```python
from build123d import *

# Parameters (mm, degrees)
SKETCH1_W               = 28
SKETCH1_H               = 16
SKETCH1_W_2             = 22.6
SKETCH1_H_2             = 11.84
BOSS_EXTRUDE1_DEPTH     = 3
BOSS_EXTRU_1_DEPTH      = 5
BOSS_EXTRU_1_DEPTH_BACK = 18
ESQUISSE6_R             = 2
BOSS_EXTRU_3_DEPTH      = 17.7
ESQUISSE7_R             = 1
ENL_V_MAT_EXTRU_3_DEPTH = 4
ESQUISSE8_W             = 11.84
ESQUISSE8_H             = 2.37
ENL_V_MAT_EXTRU_4_DEPTH = 10
CONG_1_R                = 1
CONG_3_R                = 5
CONG_4_R                = 2.5
BOSS_EXTRUDE2_DEPTH     = 23


with BuildPart() as part:
    # Sketch1 → Boss-Extrude1 (new body)
    with BuildSketch(Plane(origin=(0, 0, 0), x_dir=(1, 0, 0), z_dir=(0, 1, 0))):
        with Locations((14, 8)):
            Rectangle(SKETCH1_W, SKETCH1_H)
        with Locations((15.8, 8)):
            Rectangle(SKETCH1_W_2, SKETCH1_H_2, mode=Mode.SUBTRACT)
    extrude(amount=BOSS_EXTRUDE1_DEPTH)

    # Esquisse1 → Boss.-Extru.1 (add, two sides: drawn at the far end of the back side and taken through both)
    with BuildSketch(Plane.XY.offset(-BOSS_EXTRU_1_DEPTH_BACK)):
        Polygon((34.226941016, 3), (35.226941016, -1), (62.4, -1), (62.4, -4), (33.4, -4), (32.4, 0), (28, 0), (28, 3), align=None)
    extrude(amount=BOSS_EXTRU_1_DEPTH + BOSS_EXTRU_1_DEPTH_BACK)

    # Esquisse6 → Boss.-Extru.3 (add)
    with BuildSketch(Plane(origin=(0, 3, 0), x_dir=(1, 0, 0), z_dir=(0, 1, 0))):
        with Locations(Location((31.113470508, 0, 0), (0, 0, 90))):
            Circle(ESQUISSE6_R)
        with Locations(Location((31.113470508, 16, 0), (0, 0, 90))):
            Circle(ESQUISSE6_R)
    extrude(amount=BOSS_EXTRU_3_DEPTH)

    # Esquisse7 → Enlèv. mat.-Extru.3 (cut)
    with BuildSketch(Plane(origin=(0, 20.7, 0), x_dir=(1, 0, 0), z_dir=(0, 1, 0))):
        with Locations(Location((31.113470508, 16, 0), (0, 0, 270))):
            Circle(ESQUISSE7_R)
        with Locations(Location((31.113470508, 0, 0), (0, 0, 270))):
            Circle(ESQUISSE7_R)
    extrude(amount=-ENL_V_MAT_EXTRU_3_DEPTH, mode=Mode.SUBTRACT)

    # Esquisse8 → Enlèv. mat.-Extru.4 (cut)
    with BuildSketch(Plane(origin=(0, -1, 0), x_dir=(1, 0, 0), z_dir=(0, 1, 0))):
        with Locations((41.52, 12.315)):
            Rectangle(ESQUISSE8_W, ESQUISSE8_H)
    extrude(amount=-ENL_V_MAT_EXTRU_4_DEPTH, mode=Mode.SUBTRACT)

    # Congé1
    cong_1_edges = [part.edges().sort_by_distance(p)[0] for p in [
        (28, 1.5, -16),
    ]]
    fillet(cong_1_edges, radius=CONG_1_R)
    cong_1_2_edges = [part.edges().sort_by_distance(p)[0] for p in [
        (28, 1.5, -18),
    ]]
    fillet(cong_1_2_edges, radius=CONG_1_R - 0.0001)  # a hair under: the kernel refuses the full size

    # Congé3
    cong_3_edges = [part.edges().sort_by_distance(p)[0] for p in [
        (0, 1.5, 0),
        (0, 1.5, -16),
    ]]
    fillet(cong_3_edges, radius=CONG_3_R)

    # Congé4
    cong_4_edges = [part.edges().sort_by_distance(p)[0] for p in [
        (28, 1.5, 0),
    ]]
    fillet(cong_4_edges, radius=CONG_4_R)
    cong_4_2_edges = [part.edges().sort_by_distance(p)[0] for p in [
        (28, 1.5, 5),
    ]]
    fillet(cong_4_2_edges, radius=CONG_4_R - 0.0001)  # a hair under: the kernel refuses the full size

    # Sketch3 → Boss-Extrude2 (add)
    with BuildSketch(Plane.XY.offset(5)):
        with BuildLine():
            Line((62.4, -1), (62.4, -4))
            Line((62.4, -4), (79.480551105, -4))
            ThreePointArc((79.480551105, -4), (85.080447122, -1.680447122), (87.4, 3.919448895))
            Line((87.4, 3.919448895), (87.4, 5.5))
            ThreePointArc((87.4, 5.5), (85.9, 7), (84.4, 5.5))
            Line((84.4, 5.5), (84.4, 3.919448895))
            ThreePointArc((84.4, 3.919448895), (83.315910874, 0.78923852), (80.528063722, -1))
            Line((80.528063722, -1), (79.4, -1))
            Line((79.4, -1), (71.856339273, -1))
            Line((71.856339273, -1), (62.4, -1))
        make_face()
    extrude(amount=-BOSS_EXTRUDE2_DEPTH)


solid = part.part
```
Source: CAD feature listing. Evaluate the final solid. Frame: model axes, mm. A direction names the side the tool comes from. Coordinates: 2 decimals unless noted, no trailing zeros. Write each loop counter-clockwise with the first axis right and the second up, starting at its lowest first coordinate (ties: lowest second). Pieces come first, ordered by that corner, then holes. Notation, with made-up numbers: (74.25, 59.25) -> (119.25, 59.25) arc R16 ccw to (119.25, 77.25) -> close; hole circle Ø9 at (-18, -35). An arc over 180 degrees is marked (long way). Return JSON: item names as keys, results as strings. Group by question number.
1) Section query B-B, the plane y = 1.75. State how many separate pieces and enclosed holes the cut face has, plus the area to 3 significant figures.
2) Section query C-C, the plane z = -3.5. Return loops of the section in (x, y).
3) Section query A-A, the plane z = -9.5. Return loops of the section in (x, y).
4) Section query D-D, the plane y = 8. Return loops of the section in (x, z).
5) Mould query, pull axis Z, two halves, no side actions, for faces 4 (the face through (1, 2, -2)), 5 (the face through (85.02, -1.74, -6.34)), 6 (the face through (41, -2, -13.5)). Classes: +Z half, -Z half, draft (parallel to the pull), parting line (faces both ways), or undercut.
6) Contact query for flat-ended pins moving along their axis: P1, Ø6, axis at x = 73.5, z = -9.5, coming from the +Y side; P2, Ø1.9, axis at y = -2, z = -12, coming from the -X side; P3, Ø11.5, axis at x = 11.5, z = -5, coming from the +Y side; P4, Ø6, axis at x = 41, y = 4, coming from the -Z side. Output: stop coordinate, or through.
7) Set-up query: faces 1 (the face through (16, 1, -2.08)), 2 (the face through (31, 16.7, 0)), 3 (the face through (15, 1, 0)). Return all of +Z, -Z, +X, -X, +Y, -Y with unobstructed straight access to the full face (end or side cutting, diameter ignored); none if empty.
8) Ray query, line 1 along X through (y, z) = (18.55, 0); line 2 along X through (y, z) = (2.25, -3.5); line 3 along Y through (x, z) = (66, -8.75). Return the intervals inside material, ascending.
From the geometry:
{
 "1": {"separate pieces": "2", "enclosed holes": "1", "area": "393 mm²"},
 "2": {"outline": "(0.23, 0) -> (4.5, 0) -> (4.5, 3) -> (0.23, 3) -> close; (27.1, 0) -> (32.4, 0) -> (33.4, -4) -> (79.48, -4) arc R7.92 ccw to (87.4, 3.92) -> (87.4, 5.5) arc R1.5 ccw to (84.4, 5.5) -> (84.4, 3.92) arc R5.06 cw to (80.53, -1) -> (35.23, -1) -> (34.23, 3) -> (27.1, 3) -> close"},
 "3": {"outline": "(0, 0) -> (4.5, 0) -> (4.5, 3) -> (0, 3) -> close; (27.1, 0) -> (32.4, 0) -> (33.4, -4) -> (79.48, -4) arc R7.92 ccw to (87.4, 3.92) -> (87.4, 5.5) arc R1.5 ccw to (84.4, 5.5) -> (84.4, 3.92) arc R5.06 cw to (80.53, -1) -> (35.23, -1) -> (34.23, 3) -> (27.1, 3) -> close"},
 "4": {"outline": "circle Ø4 at (31.11, -16); circle Ø4 at (31.11, 0)"},
 "5": {"face 4": "+Z half", "face 5": "draft", "face 6": "undercut"},
 "6": {"P1": "y = -1", "P2": "x = 32.66", "P3": "y = 3", "P4": "through"},
 "7": {"face 1": "+Y, -Y", "face 2": "+Y", "face 3": "+Z, -X, +Y, -Y"},
 "8": {"line 1": "29.11 to 30.11, 32.11 to 33.11", "line 2": "0.23 to 4.5, 27.1 to 34.41, 84.12 to 87.22", "line 3": "-4 to -1"}
}
